```python
from build123d import *

# Parameters (mm, degrees)
SKETCH_1_R          = 50
EXTRUDE_1_DEPTH     = 3.302
SKETCH_2_R          = 4.7625
CUT_EXTRUDE_1_DEPTH = 71.787733429
SKETCH_4_R          = 10.16
CUT_EXTRUDE_3_DEPTH = 71.787733429
SKETCH_3_W          = 9.285115832
SKETCH_3_H          = 8.046477463
CUT_EXTRUDE_2_DEPTH = 71.787733429
SKETCH_8_R          = 8.89
SKETCH_8_W          = 5.08
SKETCH_8_H          = 40.64
CUT_EXTRUDE_4_DEPTH = 71.787733429
SKETCH_9_R          = 2.54
SKETCH_9_R_2        = 3.302
CUT_EXTRUDE_5_DEPTH = 71.787733429
SKETCH_10_R         = 1.905
CUT_EXTRUDE_6_DEPTH = 71.787733429


with BuildPart() as part:
    # 草图1 → 凸台-拉伸1 (new body)
    with BuildSketch(Plane.XY):
        with Locations(Location((0, 0, 0), (0, 0, 180))):
            Circle(SKETCH_1_R)
    extrude(amount=EXTRUDE_1_DEPTH)

    # 草图2 → 切除-拉伸1 (cut, through all)
    with BuildSketch(Plane.XY.offset(3.302)):
        with Locations((-17.78, 30.48)):
            Circle(SKETCH_2_R)
        with Locations((-25.4, -25.4)):
            Circle(SKETCH_2_R)
        with Locations((25.4, -25.4)):
            Circle(SKETCH_2_R)
        with Locations((17.78, 30.48)):
            Circle(SKETCH_2_R)
    extrude(amount=-CUT_EXTRUDE_1_DEPTH, mode=Mode.SUBTRACT)

    # 草图4 → 切除-拉伸3 (cut, through all)
    with BuildSketch(Plane.XY.offset(3.302)):
        Circle(SKETCH_4_R)
    extrude(amount=-CUT_EXTRUDE_3_DEPTH, mode=Mode.SUBTRACT)

    # 草图3 → 切除-拉伸2 (cut, through all)
    with BuildSketch(Plane.XY.offset(3.302)):
        with Locations((0, 53.807238732)):
            Rectangle(SKETCH_3_W, SKETCH_3_H)
    extrude(amount=-CUT_EXTRUDE_2_DEPTH, mode=Mode.SUBTRACT)

    # 草图8 → 切除-拉伸4 (cut, through all)
    with BuildSketch(Plane.XY.offset(3.302)):
        with Locations((34.544, 0)):
            Circle(SKETCH_8_R)
        with Locations((-34.544, 0)):
            Circle(SKETCH_8_R)
        with Locations((17.78, 0)):
            Rectangle(SKETCH_8_W, SKETCH_8_H)
        with Locations((-17.78, 0)):
            Rectangle(SKETCH_8_W, SKETCH_8_H)
    extrude(amount=-CUT_EXTRUDE_4_DEPTH, mode=Mode.SUBTRACT)

    # 草图9 → 切除-拉伸5 (cut, through all)
    with BuildSketch(Plane.XY.offset(3.302)):
        with Locations((-10.922, 15.24)):
            Circle(SKETCH_9_R)
        with Locations((10.922, 15.24)):
            Circle(SKETCH_9_R)
        with Locations((-10.922, -15.24)):
            Circle(SKETCH_9_R)
        with Locations((10.922, -15.24)):
            Circle(SKETCH_9_R)
        with Locations((0, 15.24)):
            Circle(SKETCH_9_R_2)
        with Locations((0, -15.24)):
            Circle(SKETCH_9_R_2)
    extrude(amount=-CUT_EXTRUDE_5_DEPTH, mode=Mode.SUBTRACT)

    # 草图10 → 切除-拉伸6 (cut, through all)
    with BuildSketch(Plane.XY.offset(3.302)):
        with Locations((0, 46.99)):
            Circle(SKETCH_10_R)
        with Locations((46.99, 0)):
            Circle(SKETCH_10_R)
        with Locations((0, -46.99)):
            Circle(SKETCH_10_R)
        with Locations((-46.99, 0)):
            Circle(SKETCH_10_R)
    extrude(amount=-CUT_EXTRUDE_6_DEPTH, mode=Mode.SUBTRACT)


solid = part.part
```
Geometry: final body of the model. Coordinates: model frame, mm. A direction names the side the tool comes from. Round coordinates to 2 decimals unless told otherwise and drop trailing zeros. Write each loop counter-clockwise with the first axis right and the second up, starting at its lowest first coordinate (ties: lowest second). Pieces come first, ordered by that corner, then holes.
Item 1: Set-up query: faces 1 (the face through (0.7, 10.3, 0)), 2 (the face through (18, -20.32, 2)). Return all of +Z, -Z, +X, -X, +Y, -Y with unobstructed straight access to the full face (end or side cutting, diameter ignored); none if empty.
Item 2: Section query D-D (x = -17.78). Return loops of the section in (y, z).
Item 3: Mould query, pull axis X, two halves, no side actions, for faces 3 (the face through (-0.716, 12.017, 1.674)), 4 (the face through (-2.133, -49.954, 1.628)), 5 (the face through (0.7, 10.3, 3.302)). Classes: +X half, -X half, draft (parallel to the pull), parting line (faces both ways), or undercut.
Item 4: Section query A-A (z = 2.8). Give the number of separate pieces and of enclosed holes in the cut face, plus the area to 3 significant figures.
Item 5: Section query B-B (x = -39). Return loops of the section in (y, z).
Item 6: Pin query (flat end, axial travel): P1, Ø16, axis at x = 34.544, y = 0, coming from the +Z side; P2, Ø1, axis at x = 18, z = 1, coming from the +Y side; P3, Ø1, axis at x = 17.5, z = 2, coming from the -Y side; P4, Ø1.7, axis at y = 2.5, z = 1, coming from the -X side. Return the tip coordinate at first contact, or that it passes through.
Item 7: Material intervals for L1, parallel to Y at x = 0, z = 1.45 (3 decimals); L2, parallel to X at y = -11, z = 1.7 (3 decimals); L3, parallel to X at y = 2, z = 1.15, sorted ascending.
Item 8: Section query C-C (y = 15.24). Return loops of the section in (x, z).
Completed:
1. face 1: -Z, +X, -X, +Y, -Y
1. face 2: +Z, -Z
2. outline: (-46.73, 0) - (-20.32, 0) - (-20.32, 3.3) - (-46.73, 3.3) - close; (20.32, 0) - (25.72, 0) - (25.72, 3.3) - (20.32, 3.3) - close; (35.24, 0) - (46.73, 0) - (46.73, 3.3) - (35.24, 3.3) - close
3. face 3: undercut
3. face 4: parting line
3. face 5: draft
4. separate pieces: 1
4. enclosed holes: 19
4. area: 6,140 mm2
5. outline: (-31.29, 0) - (-7.69, 0) - (-7.69, 3.3) - (-31.29, 3.3) - close; (7.69, 0) - (31.29, 0) - (31.29, 3.3) - (7.69, 3.3) - close
6. P1: passes through
6. P2: stops at y = 46.84
6. P3: stops at y = -47.02
6. P4: stops at x = -49.97
7. L1: y = -50 to -48.895, -45.085 to -18.542, -11.938 to -10.16, 10.16 to 11.938, 18.542 to 45.085, 48.895 to 49.784
7. L2: x = -48.775 to -20.32, -15.24 to 15.24, 20.32 to 48.775
7. L3: x = -49.96 to -43.21, -25.88 to -20.32, -15.24 to -9.96, 9.96 to 15.24, 20.32 to 25.88, 43.21 to 49.96
8. outline: (-47.62, 0) - (-20.32, 0) - (-20.32, 3.3) - (-47.62, 3.3) - close; (-15.24, 0) - (-13.46, 0) - (-13.46, 3.3) - (-15.24, 3.3) - close; (-8.38, 0) - (-3.3, 0) - (-3.3, 3.3) - (-8.38, 3.3) - close; (3.3, 0) - (8.38, 0) - (8.38, 3.3) - (3.3, 3.3) - close; (13.46, 0) - (15.24, 0) - (15.24, 3.3) - (13.46, 3.3) - close; (20.32, 0) - (47.62, 0) - (47.62, 3.3) - (20.32, 3.3) - close
